Part print with two shaded views. Sizes in mm from the minimum x, y, z corner. A direction names the side the tool comes from. Round coordinates to 2 decimals unless told otherwise and drop trailing zeros. Loops run counter-clockwise (first coordinate to the right, second up) from the corner with the lowest first, then second, coordinate; pieces in that order, holes last. Notation, with made-up numbers: (69.5, -7.5) - (101.5, -7.5) arc R8 ccw to (101.5, 0.5) - close; hole circle Ø1 at (-21.5, 79). An arc over 180 degrees is marked (long way). Write each question's results on one line, items separated by ' | '. Start each with the question number.
(1) Cut at B-B, the plane y = 10. List the corners of the cut face in (x, z), then the cut area to 4 significant figures.
(2) Mould opens along X. For the marked faces 1, 2 and 3 say: released by +X, released by -X, zero draft, split by the parting line, or undercut.
(3) Drill centre lines: L1, parallel to Y at x = 11.4, z = 20; L2, parallel to X at y = 23.25, z = 5; L3, parallel to Y at x = 10.5, z = 4.25. Where is each one in solid material? Low to high.
(4) Cut at A-A, the plane z = 5. List the corners of the cut face in (x, y), then the cut area to 3 significant figures.
(5) Cut at D-D, the plane x = 17. List the corners of the cut face in (y, z).
(6) Flat gauge pins, fed straight in: P1, Ø10, axis at x = 23.5, z = 7, coming from the +Y side; P2, Ø10, axis at x = 13.5, y = 15.5, coming from the +Z side; P3, Ø2.5, axis at y = 3.5, z = 20, coming from the +X side; P4, Ø4, axis at x = 7, y = 6.5, coming from the -Z side. Where does each tip first touch, or does it go through?
(7) Cut at C-C, the plane x = 36. List the corners of the cut face in (y, z).
(8) Tool access for the marked faces 4, 5, 6 and 7: list every direction of +Z, -Z, +X, -X, +Y, -Y with a clear straight run to the whole face (end or side of a thin tool).
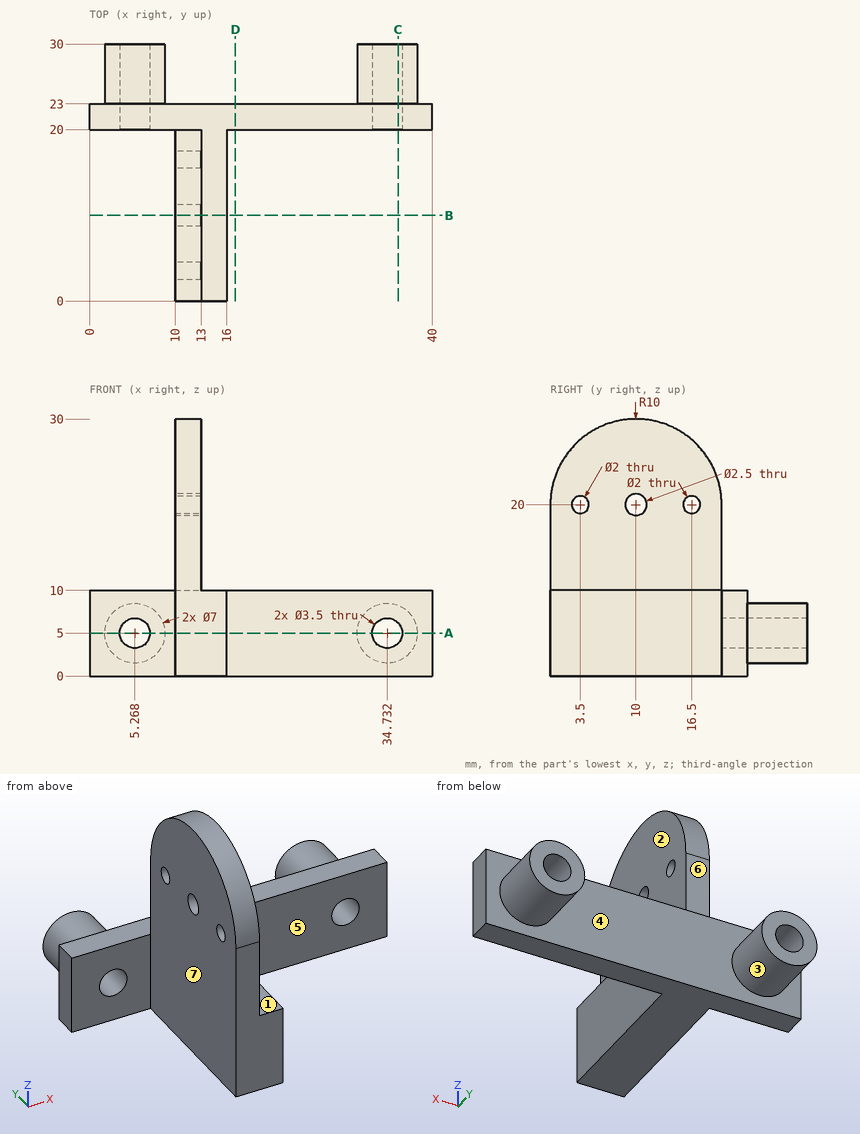
A:
1) outline: (10, 0) - (16, 0) - (16, 10) - (13, 10) - (13, 18.75) - (10, 18.75) - close; (10, 21.25) - (13, 21.25) - (13, 30) - (10, 30) - close | area: 112.5 mm2
2) face 1: zero draft | face 2: released by +X | face 3: undercut
3) L1: 0 to 2.5, 4.5 to 8.75, 11.25 to 15.5, 17.5 to 20 | L2: 1.77 to 3.52, 7.02 to 8.77, 31.23 to 32.98, 36.48 to 38.23 | L3: 0 to 23
4) outline: (0, 20) - (3.52, 20) - (3.52, 30) - (1.77, 30) - (1.77, 23) - (0, 23) - close; (7.02, 20) - (10, 20) - (10, 0) - (16, 0) - (16, 20) - (32.98, 20) - (32.98, 30) - (31.23, 30) - (31.23, 23) - (8.77, 23) - (8.77, 30) - (7.02, 30) - close; (36.48, 20) - (40, 20) - (40, 23) - (38.23, 23) - (38.23, 30) - (36.48, 30) - close | area: 268 mm2
5) outline: (20, 0) - (23, 0) - (23, 10) - (20, 10) - close
6) P1: y = 23 | P2: z = 29.99 | P3: x = 13 | P4: through
7) outline: (20, 0) - (23, 0) - (23, 1.74) - (30, 1.74) - (30, 3.79) - (20, 3.79) - close; (20, 6.21) - (30, 6.21) - (30, 8.26) - (23, 8.26) - (23, 10) - (20, 10) - close
8) face 4: +Y | face 5: +Z, -Z, +X, -Y | face 6: +Z, +X, -X, +Y | face 7: +Z, -Z, -X, -Y
